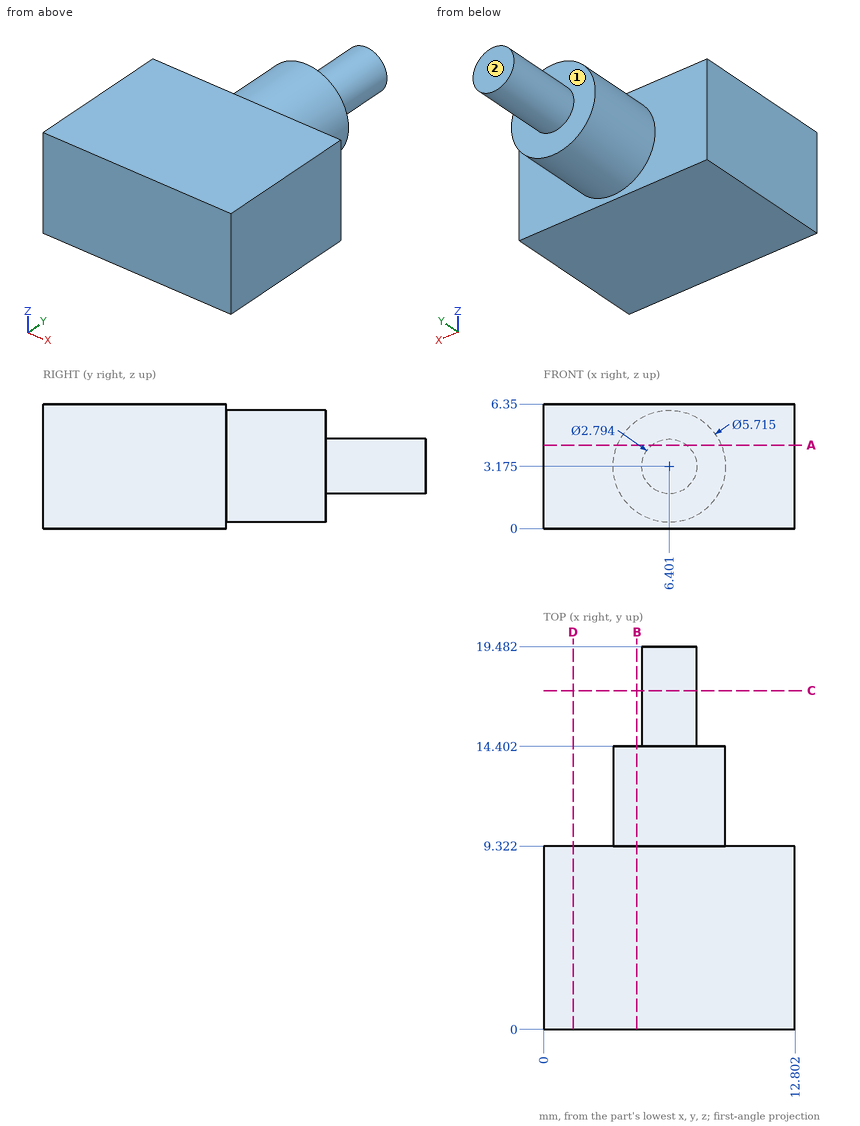
For this review, use the dimensioned drawing (mm, ordinates from the lowest corner) and the shaded views. A direction names the side the tool comes from. Give positions to 0.01 mm unless a question says otherwise; leave off trailing zeros. Order: outer loops, then holes, each group sorted by start corner. A loop starts at its lowest first (then second) coordinate and runs counter-clockwise, first axis right, second up. Notation, with made-up numbers: (-25.5, 41) - (-20.5, 41) arc R18 cw to (-20.5, 50) - close; hole circle Ø2 at (-29, 10). An arc over 180 degrees is marked (long way). Use CSV: the item, a comma, the result in double quotes. Start each with the question number.
Q1. Take a section at A-A (z = 4.25). State the section outline as (x, y) points.
Q2. For P1, Ø3, axis at y = 16.5, z = 1.5, coming from the +X side; P2, Ø1, axis at y = 10.5, z = 3.5, coming from the +X side; P3, Ø1.5, axis at y = 16, z = 3.5, coming from the -X side, all flat-tipped, find the tip position at first contact; note any pin that passes through.
Q3. Machinability: for the marked faces 1 and 2, which of the approach directions +Z, -Z, +X, -X, +Y, -Y give a long, thin tool a straight path to every point of the face, cutting with its end or side? Answer none if there is none.
Q4. For line 1 (Y direction, x = 1, z = 4.5); line 2 (Y direction, x = 8, z = 2); line 3 (X direction, y = 18.25, z = 3.25) (1 decimal), list the stretches that pass through material, from the lowest coordinate up.
Q5. Take a section at B-B (x = 4.75). State the section outline as (y, z) points.
Q6. Take a section at C-C (y = 17.25). State the section outline as (x, z) points (1 decimal).
Q7. Take a section at D-D (x = 1.5). State the section outline as (y, z) points.
Calculated:
1,outline,"(0, 0) - (12.8, 0) - (12.8, 9.32) - (9.05, 9.32) - (9.05, 14.4) - (7.29, 14.4) - (7.29, 19.48) - (5.51, 19.48) - (5.51, 14.4) - (3.75, 14.4) - (3.75, 9.32) - (0, 9.32) - close"
2,P1,"stops at x = 7.79"
2,P2,"stops at x = 9.26"
2,P3,"stops at x = 5"
3,face 1,"+Y"
3,face 2,"+Z, -Z, +X, -X, +Y"
4,line 1,"y = 0 to 9.32"
4,line 2,"y = 0 to 14.4"
4,line 3,"x = 5 to 7.8"
5,outline,"(0, 0) - (9.32, 0) - (9.32, 0.84) - (14.4, 0.84) - (14.4, 5.51) - (9.32, 5.51) - (9.32, 6.35) - (0, 6.35) - close"
6,outline,"circle Ø2.8 at (6.4, 3.2)"
7,outline,"(0, 0) - (9.32, 0) - (9.32, 6.35) - (0, 6.35) - close"
